```python
from build123d import *

# Parameters (mm, degrees)
SKETCH1_R           = 34.445
BOSS_EXTRUDE1_DEPTH = 22
SKETCH15_R          = 34.445
CUT_EXTRUDE2_DEPTH  = 54.450126754
CUT_EXTRUDE4_START  = -1
SKETCH17_R          = 6.2
CUT_EXTRUDE4_DEPTH  = 20
SKETCH18_R          = 7.25
CUT_EXTRUDE5_DEPTH  = 41.489614217
SKETCH19_R          = 6.25
CUT_EXTRUDE7_DEPTH  = 21
SKETCH20_R          = 9.845995641
CUT_EXTRUDE9_DEPTH  = 10
FILLET12_R          = 6
SKETCH23_R          = 4
SKETCH23_R_2        = 2
CUT_EXTRUDE10_DEPTH = 41.489614217
CUT_EXTRUDE11_START = -12
CUT_EXTRUDE11_DEPTH = 29.489614217
FILLET19_R          = 3
SKETCH25_R          = 11
CUT_EXTRUDE12_DEPTH = 10
FILLET20_R          = 2


with BuildPart() as part:
    # Sketch1 → Boss-Extrude1 (new body)
    with BuildSketch(Plane(origin=(0, 0, 0), x_dir=(1, 0, 0), z_dir=(0, 1, 0))):
        with Locations(Location((0, 0, 0), (0, 0, 270))):
            Circle(SKETCH1_R)
    extrude(amount=BOSS_EXTRUDE1_DEPTH)

    # Sketch15 → Cut-Extrude2 (cut, through all)
    with BuildSketch(Plane(origin=(0, 22, 0), x_dir=(1, 0, 0), z_dir=(0, 1, 0))):
        Circle(SKETCH15_R)
        with BuildLine():
            Line((-19.109582045, 20.616901016), (-19.109582045, -17.678671312))
            Line((-19.109582045, -17.678671312), (19.109582045, -17.678671312))
            Line((19.109582045, -17.678671312), (19.109582045, 20.616901016))
            ThreePointArc((19.109582045, 20.616901016), (0, 28.111078483), (-19.109582045, 20.616901016))
        make_face(mode=Mode.SUBTRACT)
    extrude(amount=-CUT_EXTRUDE2_DEPTH, mode=Mode.SUBTRACT)

    # Sketch17 → Cut-Extrude4 (cut)
    with BuildSketch(Plane(origin=(0, 22, 0), x_dir=(1, 0, 0), z_dir=(0, 1, 0)).offset(CUT_EXTRUDE4_START)):
        with Locations(Location((-11.644122412, -9.008465082, 0), (0, 0, 270))):
            Circle(SKETCH17_R)
        with Locations(Location((11.644122412, -9.008465082, 0), (0, 0, 90))):
            Circle(SKETCH17_R)
    extrude(amount=-CUT_EXTRUDE4_DEPTH, mode=Mode.SUBTRACT)

    # Sketch18 → Cut-Extrude5 (cut, through all)
    with BuildSketch(Plane(origin=(0, 22, 0), x_dir=(1, 0, 0), z_dir=(0, 1, 0))):
        with Locations(Location((0, 5.846291401, 0), (0, 0, 270))):
            Circle(SKETCH18_R)
    extrude(amount=-CUT_EXTRUDE5_DEPTH, mode=Mode.SUBTRACT)

    # Sketch19 → Cut-Extrude7 (cut)
    with BuildSketch(Plane(origin=(0, 22, 0), x_dir=(1, 0, 0), z_dir=(0, 1, 0))):
        with Locations((0, 22.497935332)):
            Circle(SKETCH19_R)
    extrude(amount=-CUT_EXTRUDE7_DEPTH, mode=Mode.SUBTRACT)

    # Sketch20 → Cut-Extrude9 (cut)
    with BuildSketch(Plane(origin=(0, 22, 0), x_dir=(1, 0, 0), z_dir=(0, 1, 0))):
        with Locations(Location((0, 5.846291401, 0), (0, 0, 270))):
            Circle(SKETCH20_R)
    extrude(amount=-CUT_EXTRUDE9_DEPTH, mode=Mode.SUBTRACT)

    # Fillet12
    fillet12_edges = [part.edges().sort_by_distance(p)[0] for p in [
        (-19.109582045, 11, 17.678671312),
        (19.109582045, 11, 17.678671312),
    ]]
    fillet(fillet12_edges, radius=FILLET12_R)

    # Sketch23 → Cut-Extrude10 (cut, through all)
    with BuildSketch(Plane(origin=(0, 22, 0), x_dir=(1, 0, 0), z_dir=(0, 1, 0))):
        with Locations(Location((-11.644122412, -9.008465082, 0), (0, 0, 270))):
            Circle(SKETCH23_R)
        with Locations(Location((11.644122412, -9.008465082, 0), (0, 0, 270))):
            Circle(SKETCH23_R)
        with Locations(Location((0, -9.008465082, 0), (0, 0, 270))):
            Circle(SKETCH23_R_2)
    extrude(amount=-CUT_EXTRUDE10_DEPTH, mode=Mode.SUBTRACT)

    # Sketch24 → Cut-Extrude11 (cut, through all)
    with BuildSketch(Plane.XZ.offset(CUT_EXTRUDE11_START)):
        with BuildLine():
            Line((-19.109582045, -20.616901016), (-19.109582045, 2.30978602))
            Line((-19.109582045, 2.30978602), (19.109582045, 2.30978602))
            Line((19.109582045, 2.30978602), (19.109582045, -20.616901016))
            ThreePointArc((19.109582045, -20.616901016), (0, -28.111078483), (-19.109582045, -20.616901016))
        make_face()
    extrude(amount=-CUT_EXTRUDE11_DEPTH, mode=Mode.SUBTRACT)

    # Fillet19
    fillet19_edges = [part.edges().sort_by_distance(p)[0] for p in [
        (-19.109582045, 17, 2.30978602),
        (12.31259954, 12, 2.30978602),
        (-12.31259954, 12, 2.30978602),
        (-19.109582045, 12, -9.153557498),
        (19.109582045, 12, -9.153557498),
        (19.109582045, 17, 2.30978602),
    ]]
    fillet(fillet19_edges, radius=FILLET19_R)

    # Sketch25 → Cut-Extrude12 (cut)
    with BuildSketch(Plane(origin=(0, 12, 0), x_dir=(1, 0, 0), z_dir=(0, 1, 0))):
        with Locations((0, 5.846291401)):
            Circle(SKETCH25_R)
    extrude(amount=-CUT_EXTRUDE12_DEPTH, mode=Mode.SUBTRACT)

    # Fillet20
    fillet20_edges = [part.edges().sort_by_distance(p)[0] for p in [
        (2.158391198, 7, -16.632456031),
        (-2.158391198, 7, -16.632456031),
    ]]
    fillet(fillet20_edges, radius=FILLET20_R)


solid = part.part
```
Geometry check sheet. Reference: the model listing, model coordinates, mm. A direction names the side the tool comes from. Give positions to 0.01 mm unless a question says otherwise; leave off trailing zeros. Order: outer loops, then holes, each group sorted by start corner. A loop starts at its lowest first (then second) coordinate and runs counter-clockwise, first axis right, second up. Notation, with made-up numbers: (16.25, 78) - (55.25, 78) arc R19 ccw to (55.25, 102) - close; hole circle Ø7 at (-3.5, 52). An arc over 180 degrees is marked (long way). Answer in a Markdown table with one row per item. Add a question column.
Q1. Material ranges on probe 1 along X at (y, z) = (14, 8.5) (3 decimals); probe 2 along Z at (x, y) = (-8, 11); probe 3 along Y at (x, z) = (2.5, 1), recorded low to high. Write a range as from..to.
Q2. Mould release check, pull along X, two halves, no side actions. Record for faces 4 (the cylindrical face through (-17.399, 10.846, 15.874)), 5 (the flat face through (0, 1, -22)), 6 (the flat face through (0, 22, 12)): pulls with the +X half, pulls with the -X half, needs draft (parallel to the pull), parting line crosses it, or undercut.
Q3. Cross-section at B-B, the plane z = -2.5. Enter the section's corners in (x, y).
Q4. Gauge pin test, flat ends, axial feed: pin 1 (8 mm diameter, centred on x = 9.5, z = 8, fed in from -Y); pin 2 (1 mm diameter, centred on y = 10, z = -5, fed in from -X); pin 3 (9.5 mm diameter, centred on x = 0.5, z = -19.5, fed in from +Y); pin 4 (6.5 mm diameter, centred on x = -2, z = -12, fed in from +Y). Record the tip position at first contact, or that the pin passes through.
Q5. Tool access check on faces 1 (the cylindrical face through (18.21, 11.14, -12.02)), 2 (the flat face through (11, 18, 2.31)), 3 (the cylindrical face through (9.782, 11.14, 3.095)). Record the directions out of +Z, -Z, +X, -X, +Y, -Y that give a thin tool (end or side, any length) a straight path to the whole face; none if there is none.
Q6. Cross-section at A-A, the plane x = 0. Enter the section's corners in (y, z).
Q7. Cross-section at C-C, the plane y = 14. Count the separate pieces of the cut face and the enclosed holes in it, then the cut area to 3 significant figures.
Check values:
| question | item | result |
|---|---|---|
| 1 | probe 1 | x = -19.11..-17.823, -5.465..-1.934, 1.934..5.465, 17.823..19.11 |
| 1 | probe 2 | z = -26.95..-13.4, 1.7..3.99, 14.02..17.68 |
| 1 | probe 3 | y = 0..2 |
| 2 | face 4 | pulls with the -X half |
| 2 | face 5 | undercut |
| 2 | face 6 | needs draft |
| 3 | outline | (-19.11, 0) - (-6.43, 0) - (-6.43, 2) - (-10.48, 2) - (-10.48, 12) - (-16.11, 12) arc R3 ccw to (-19.11, 9) - close; (6.43, 0) - (19.11, 0) - (19.11, 9) arc R3 ccw to (16.11, 12) - (10.48, 12) - (10.48, 2) - (6.43, 2) - close |
| 4 | pin 1 | stops at y = 0 |
| 4 | pin 2 | stops at x = -19.07 |
| 4 | pin 3 | stops at y = 12 |
| 4 | pin 4 | stops at y = 2 |
| 5 | face 1 | -Z, +X, +Y |
| 5 | face 2 | -Z, +X, -X, +Y |
| 5 | face 3 | none |
| 6 | outline | (0, -28.11) - (1, -28.11) - (1, -16.25) - (2, -16.25) - (2, -13.1) - (0, -13.1) - close; (0, 1.4) - (2, 1.4) - (2, 5.15) - (12, 5.15) - (12, 4) - (22, 4) - (22, 7.01) - (0, 7.01) - close; (0, 11.01) - (22, 11.01) - (22, 17.68) - (0, 17.68) - close |
| 7 | separate pieces | 1 |
| 7 | enclosed holes | 3 |
| 7 | area | 306 mm^2 |
